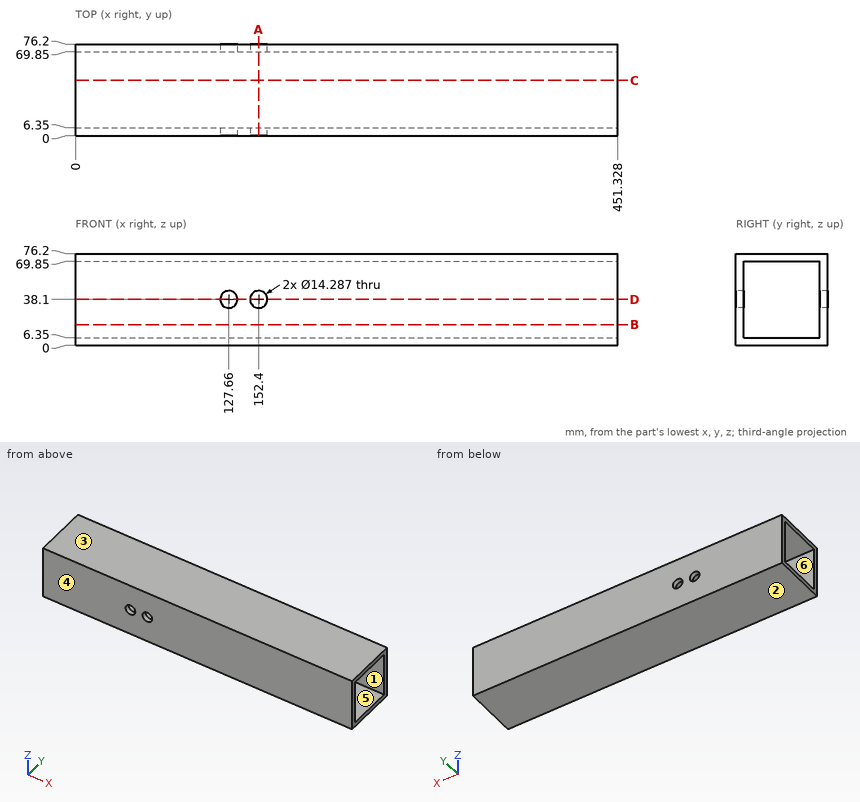
Drawing for the job (mm, zero at the part's lowest x, y, z). A direction names the side the tool comes from. Round coordinates to 2 decimals unless told otherwise and drop trailing zeros. Write each loop counter-clockwise with the first axis right and the second up, starting at its lowest first coordinate (ties: lowest second). Pieces come first, ordered by that corner, then holes.
Item 1: Band-saw the part on A-A on x = 152.4. Write the cut outline in (y, z), then the cut area to 3 significant figures.
Filled in:
outline: (0, 0) - (76.2, 0) - (76.2, 30.96) - (69.85, 30.96) - (69.85, 6.35) - (6.35, 6.35) - (6.35, 30.96) - (0, 30.96) - close; (0, 45.24) - (6.35, 45.24) - (6.35, 69.85) - (69.85, 69.85) - (69.85, 45.24) - (76.2, 45.24) - (76.2, 76.2) - (0, 76.2) - close
area: 1,590 mm2
Item 2: Tool access for the marked faces 1 and 2: list every direction of +Z, -Z, +X, -X, +Y, -Y with a clear straight run to the whole face (end or side of a thin tool).
Filled in:
face 1: +X, -X
face 2: -Z, +X, -X, +Y, -Y
Item 3: Mould opens along Y. For the marked faces 3, 4, 5 and 6 say: released by +Y, released by -Y, zero draft, split by the parting line, or undercut.
Filled in:
face 3: zero draft
face 4: released by -Y
face 5: undercut
face 6: undercut
Item 4: Drill centre lines: L1, parallel to X at y = 72, z = 38; L2, parallel to Y at x = 282.5, z = 38. Where is each one in solid material? Low to high.
Filled in:
L1: x = 0 to 120.52, 134.8 to 145.26, 159.54 to 451.33
L2: y = 0 to 6.35, 69.85 to 76.2
Item 5: Band-saw the part on D-D on z = 38.1. Give the number of separate pieces and of enclosed holes in the cut face, then the cut area to 3 significant figures.
Filled in:
separate pieces: 6
enclosed holes: 0
area: 5,370 mm2
Item 6: Band-saw the part on B-B on z = 17. Write the cut outline in (x, y), then the cut area to 3 significant figures.
Filled in:
outline: (0, 0) - (451.33, 0) - (451.33, 6.35) - (0, 6.35) - close; (0, 69.85) - (451.33, 69.85) - (451.33, 76.2) - (0, 76.2) - close
area: 5,730 mm2
Item 7: Drop a flat-ended pin along its axis: pin 1 Ø23 at (x, z) = (127.66, 38.1) entering from +Y. Give the stop position or say it passes through.
Filled in:
pin 1: stops at y = 76.2
